```python
from build123d import *

# Parameters (mm, degrees)
EXTRUS_O1_DEPTH = 9.3
EXTRUS_O2_DEPTH = 7.3
ESCALA3_SCALE   = 1.05
ESBO_O3_R       = 30
EXTRUS_O3_DEPTH = 8
ESBO_O4_R       = 2.5
EXTRUS_O6_DEPTH = 8


with BuildPart() as part:
    # Esboço1 → Extrusão1 (new body)
    with BuildSketch(Plane(origin=(0, 0, 0), x_dir=(1, 0, 0), z_dir=(0, 1, 0))):
        with BuildLine():
            Line((3.9, 0), (0, 0))
            Line((0, 0), (-3.9, 0))
            Line((-3.9, 0), (-3.9, -2.711549373))
            ThreePointArc((-3.9, -2.711549373), (0, -4.75), (3.9, -2.711549373))
            Line((3.9, -2.711549373), (3.9, 0))
        make_face()
        with BuildLine():
            Line((-3.9, 0), (0, 0))
            Line((0, 0), (3.9, 0))
            Line((3.9, 0), (3.9, 2.711549373))
            ThreePointArc((3.9, 2.711549373), (0, 4.75), (-3.9, 2.711549373))
            Line((-3.9, 2.711549373), (-3.9, 0))
        make_face()
        with BuildLine():
            Line((-3.9, 0), (0, 0))
            Line((0, 0), (3.9, 0))
            Line((3.9, 0), (3.9, 2.711549373))
            ThreePointArc((3.9, 2.711549373), (0, 4.75), (-3.9, 2.711549373))
            Line((-3.9, 2.711549373), (-3.9, 0))
        make_face()
    extrude(amount=EXTRUS_O1_DEPTH)

    # Esboço2 → Extrusão2 (cut)
    with BuildSketch(Plane(origin=(0, 9.3, 0), x_dir=(1, 0, 0), z_dir=(0, 1, 0))):
        with BuildLine():
            Line((-1.9, 0), (0, 0))
            Line((0, 0), (1.9, 0))
            Line((1.9, 0), (1.9, 1.988089535))
            ThreePointArc((1.9, 1.988089535), (0, 2.75), (-1.9, 1.988089535))
            Line((-1.9, 1.988089535), (-1.9, 0))
        make_face()
        with BuildLine():
            Line((1.9, 0), (0, 0))
            Line((0, 0), (-1.9, 0))
            Line((-1.9, 0), (-1.9, -1.988089535))
            ThreePointArc((-1.9, -1.988089535), (0, -2.75), (1.9, -1.988089535))
            Line((1.9, -1.988089535), (1.9, 0))
        make_face()
    extrude(amount=-EXTRUS_O2_DEPTH, mode=Mode.SUBTRACT)


with BuildPart() as part_1:
    # Escala3: scaled about (0, 0, 0)
    add(part.part.scale(ESCALA3_SCALE))

    # Esboço3 → Extrusão3 (add)
    with BuildSketch(Plane.XZ):
        with Locations(Location((0, 0, 0), (0, 0, 270))):
            Circle(ESBO_O3_R)
    extrude(amount=EXTRUS_O3_DEPTH)

    # Varredura de corte1: sweep along a path in Esboço6
    with BuildLine(Plane(origin=(0, -4, 0), x_dir=(-1, 0, 0), z_dir=(0, 1, 0))) as varredura_de_corte1_path:
        CenterArc((0, 0), 30, 0, 360)
    # Esboço4 → Varredura de corte1 (sweep, cut)
    with BuildSketch(Plane(origin=(0, 0, 0), x_dir=(0, 0, -1), z_dir=(1, 0, 0))):
        with Locations((-30, -4)):
            Circle(ESBO_O4_R)
    sweep(path=varredura_de_corte1_path.line, mode=Mode.SUBTRACT)

    # Esboço7 → Extrusão6 (cut)
    with BuildSketch(Plane.XZ.offset(8)):
        with BuildLine():
            Line((-21.650635095, 12.5), (-5.629165125, 3.25))
            ThreePointArc((-5.629165125, 3.25), (-3.25, 5.629165125), (0, 6.5))
            Line((0, 6.5), (0, 25))
            ThreePointArc((0, 25), (-12.5, 21.650635095), (-21.650635095, 12.5))
        make_face()
        with BuildLine():
            Line((0, -25), (0, -6.5))
            ThreePointArc((0, -6.5), (-3.25, -5.629165125), (-5.629165125, -3.25))
            Line((-5.629165125, -3.25), (-21.650635095, -12.5))
            ThreePointArc((-21.650635095, -12.5), (-12.5, -21.650635095), (0, -25))
        make_face()
        with BuildLine():
            Line((21.650635095, 12.5), (5.629165125, 3.25))
            ThreePointArc((5.629165125, 3.25), (6.5, 0), (5.629165125, -3.25))
            Line((5.629165125, -3.25), (21.650635095, -12.5))
            ThreePointArc((21.650635095, -12.5), (25, 0), (21.650635095, 12.5))
        make_face()
    extrude(amount=-EXTRUS_O6_DEPTH, mode=Mode.SUBTRACT)


solid = part_1.part
```
Design review of the part built by this model. Coordinates are the model's own, in mm. A direction names the side the tool comes from. Give positions to 0.01 mm unless a question says otherwise; leave off trailing zeros. Loops run counter-clockwise (first coordinate to the right, second up) from the corner with the lowest first, then second, coordinate; pieces in that order, holes last. Notation, with made-up numbers: M 29,-13 L 74,-13 A22 ccw 74,21 Z; hole C -23,-20.75 d3. An arc over 180 degrees is marked long. Return JSON: item names as keys, results as strings. Group by question number.
Item 1: We need section B-B (z = 0). Give the boundary of the cut face in (x, y) (3 decimals).
Item 2: We need section A-A (y = 8). Give the boundary of the cut face in (x, z) (1 decimal), and give its area (3 significant figures).
Item 3: We need section C-C (y = -3.25). Give the boundary of the cut face in (x, z), and give its area (3 significant figures).
Item 4: We need section D-D (x = -13.5). Give the number of separate pieces and of enclosed holes in the cut face, and give its area (3 significant figures).
Item 5: For probe 1 along X at (y, z) = (-0.75, 11); probe 2 along X at (y, z) = (-0.75, -7.5); probe 3 along Z at (x, y) = (-10.5, -5.25), list the stretches that pass through material, from the lowest coordinate up.
Item 6: Tool access review of faces 1 (the cylindrical face through (0.067, 4.814, -4.987)), 2 (the cylindrical face through (-12.34, -4.06, 21.74)), 3 (the flat face through (-1.995, 6, 0)), 4 (the flat face through (0, -8, 0)): name each direction out of +Z, -Z, +X, -X, +Y, -Y from which nothing blocks a thin tool from reaching the whole face with its end or side.
Item 7: Insertion check: pin 1 Ø1 at (x, z) = (16, 9) entering from +Y; pin 2 Ø2 at (x, y) = (-1, 4) entering from +Z; pin 3 Ø2 at (y, z) = (7.5, 0) entering from -X (3 decimals). Each pin has a flat end and moves straight along its axis. Give the tip position at first contact, or say it passes through.
Item 8: Mouldability with a two-part tool opening along Z and no side actions: class faces 5 (the cylindrical face through (-0.067, 4.814, 4.987)), 6 (the flat face through (-4.095, 5, 0)), 7 (the cylindrical face through (0.031, 5.986, -2.887)) as released by +Z, released by -Z, zero draft, split by the parting line, or undercut.
Output:
{
 "1": {"outline": "M -30,-8 L 6.5,-8 L 6.5,0 L 4.095,0 L 4.095,9.765 L 1.995,9.765 L 1.995,2.1 L -1.995,2.1 L -1.995,9.765 L -4.095,9.765 L -4.095,0 L -30,0 L -30,-1.5 A2.5 cw -30,-6.5 Z; M 25,-8 L 30,-8 L 30,-6.5 A2.5 cw 30,-1.5 L 30,0 L 25,0 Z"},
 "2": {"outline": "M -4.1,-2.8 A5 ccw 4.1,-2.8 L 4.1,2.8 A5 ccw -4.1,2.8 Z; hole M -2,-2.1 A2.9 ccw 2,-2.1 L 2,2.1 A2.9 ccw -2,2.1 Z", "area": "50.2 mm^2"},
 "3": {"outline": "C 0,0 d55.23; hole M -21.65,-12.5 A25 ccw 0,-25 L 0,-6.5 A6.5 cw -5.63,-3.25 Z; hole M -21.65,12.5 L -5.63,3.25 A6.5 cw 0,6.5 L 0,25 A25 ccw Z; hole M 5.63,-3.25 L 21.65,-12.5 A25 ccw 21.65,12.5 L 5.63,3.25 A6.5 cw Z", "area": "1,480 mm^2"},
 "4": {"separate pieces": "3", "enclosed holes": "0", "area": "194 mm^2"},
 "5": {"probe 1": "x = -27.91 to -19.05, 0 to 19.05, 22.45 to 27.91", "probe 2": "x = -29.05 to -12.99, 0 to 12.99, 23.85 to 29.05", "probe 3": "z = -25.78 to -22.69, -6.06 to 6.06, 22.69 to 25.78"},
 "6": {"face 1": "-Z, +Y", "face 2": "+Y, -Y", "face 3": "+Y", "face 4": "+Z, -Z, +X, -X, -Y"},
 "7": {"pin 1": "stops at y = 0", "pin 2": "stops at z = 4.99", "pin 3": "stops at x = -4.095"},
 "8": {"face 5": "released by +Z", "face 6": "zero draft", "face 7": "undercut"}
}
